Check sheet for the modelled part. Datum: model origin and axes. Units: mm. Face numbers are marked on the shaded views. A direction names the side the tool comes from. Round coordinates to 2 decimals unless told otherwise and drop trailing zeros. Order: outer loops, then holes, each group sorted by start corner. A loop starts at its lowest first (then second) coordinate and runs counter-clockwise, first axis right, second up.
```python
from build123d import *

# Parameters (mm, degrees)
BOX031_W                 = 46
BOX031_H                 = 15
BOX031_DEPTH             = 16
BOX029_W                 = 78
BOX029_H                 = 15
BOX029_DEPTH             = 6
BOX023_W                 = 220
BOX023_H                 = 2.5
BOX023_DEPTH             = 3
EXTRUDE011_DEPTH         = 10
BOX024_W                 = 220
BOX024_H                 = 113
BOX024_DEPTH             = 8
BOX026_W                 = 32
BOX026_H                 = 6
BOX026_DEPTH             = 6
PRISM004_DEPTH           = 6
PRISM004_PLACEMENT_ANGLE = 30
PRISM005_DEPTH           = 6
PRISM005_PLACEMENT_ANGLE = 30
EXTRUDE012_DEPTH         = 12.5
EXTRUDE009_DEPTH         = 12.5
EXTRUDE008_DEPTH         = 12.5
BOX009_W                 = 12.5
BOX009_H                 = 7.5
BOX009_DEPTH             = 22
BOX010_W                 = 12.5
BOX010_H                 = 7.5
BOX010_DEPTH             = 22
CYLINDER_R               = 1.7
CYLINDER_DEPTH           = 30
BOX007_W                 = 15
BOX007_H                 = 70
BOX007_DEPTH             = 6
BOX006_W                 = 40
BOX006_H                 = 51
BOX006_DEPTH             = 6
EXTRUDE010_DEPTH         = 12.5
BOX021_W                 = 12.5
BOX021_H                 = 7.5
BOX021_DEPTH             = 22
BOX027_W                 = 12.5
BOX027_H                 = 7.5
BOX027_DEPTH             = 22
CYLINDER002_R            = 1.7
CYLINDER002_DEPTH        = 30
BOX025_W                 = 15
BOX025_H                 = 70
BOX025_DEPTH             = 6
BOX022_W                 = 40
BOX022_H                 = 51
BOX022_DEPTH             = 6
BOX005_W                 = 20
BOX005_H                 = 6
BOX005_DEPTH             = 30
BOX004_W                 = 40
BOX004_H                 = 6
BOX004_DEPTH             = 44.5


with BuildPart() as cube030:
    # Box031 → Box031 (new body)
    with BuildSketch(Plane(origin=(-22, 15, 0), x_dir=(1, 0, 0), z_dir=(0, 0, 1))):
        with Locations((23, 7.5)):
            Rectangle(BOX031_W, BOX031_H)
    extrude(amount=BOX031_DEPTH)


with BuildPart() as cube028:
    # Box029 → Box029 (new body)
    with BuildSketch(Plane(origin=(-39, 0, 0), x_dir=(1, 0, 0), z_dir=(0, 0, 1))):
        with Locations((39, 7.5)):
            Rectangle(BOX029_W, BOX029_H)
    extrude(amount=BOX029_DEPTH)


with BuildPart() as cube022:
    # Box023 → Box023 (new body)
    with BuildSketch(Plane(origin=(-110, 2, 0), x_dir=(1, 0, 0), z_dir=(0, 0, 1))):
        with Locations((110, 1.25)):
            Rectangle(BOX023_W, BOX023_H)
    extrude(amount=BOX023_DEPTH)


with BuildPart() as extrude011:
    # Sketch009 → Extrude011 (new body)
    with BuildSketch(Plane.XY):
        Polygon((-95, 0), (95, 0), (85, 61), (-85, 61), align=None)
    extrude(amount=EXTRUDE011_DEPTH)


with BuildPart() as obj1:
    # Box024 → Box024 (new body)
    with BuildSketch(Plane(origin=(-110, -15, 0), x_dir=(1, 0, 0), z_dir=(0, 0, 1))):
        with Locations((110, 56.5)):
            Rectangle(BOX024_W, BOX024_H)
    extrude(amount=BOX024_DEPTH)

    # Cut004020: cut Extrude011
    add(extrude011.part, mode=Mode.SUBTRACT)


with BuildPart() as cube025:
    # Box026 → Box026 (new body)
    with BuildSketch(Plane(origin=(-16, 55, 0), x_dir=(1, 0, 0), z_dir=(0, 0, 1))):
        with Locations((16, 3)):
            Rectangle(BOX026_W, BOX026_H)
    extrude(amount=BOX026_DEPTH)


with BuildPart() as prism004:
    # Prism004 → Prism004 (new body)
    with BuildSketch(Plane.XY):
        Polygon((45, 0), (-22.5, 38.971143), (-22.5, -38.971143), align=None)
    extrude(amount=PRISM004_DEPTH)


with BuildPart() as prism004_1:
    # Prism004 placement: moved
    add(prism004.part.moved(Location((0, 23, 0))).rotate(Axis((0, 23, 0), (0, 0, -1)), PRISM004_PLACEMENT_ANGLE))


with BuildPart() as obj2:
    # Prism005 → Prism005 (new body)
    with BuildSketch(Plane.XY):
        Polygon((60, 0), (-30, 51.961524), (-30, -51.961524), align=None)
    extrude(amount=PRISM005_DEPTH)


with BuildPart() as obj2_1:
    # Prism005 placement: moved
    add(obj2.part.moved(Location((0, 23, 0))).rotate(Axis((0, 23, 0), (0, 0, -1)), PRISM005_PLACEMENT_ANGLE))

    # Cut004019: cut Prism004
    add(prism004_1.part, mode=Mode.SUBTRACT)


with BuildPart() as obj2_2:
    # Cut004019 placement: moved
    add(obj2_1.part.moved(Location((0, 7, 0))))

    # Fusion004005: union Cube025
    add(cube025.part)

    # Cut004015: cut obj1
    add(obj1.part, mode=Mode.SUBTRACT)

    # Cut004016: cut Cube022
    add(cube022.part, mode=Mode.SUBTRACT)


with BuildPart() as extrude012:
    # Sketch010 (on Face21 of Fusion004006) → Extrude012 (new body)
    with BuildSketch(Plane(origin=(-20, 0, 0), x_dir=(0, -1, 0), z_dir=(-1, 0, 0))):
        Polygon((-7.5, 0), (-7.5, 25), (-21.933757, 0), align=None)
    extrude(amount=-EXTRUDE012_DEPTH)


with BuildPart() as extrude012_1:
    # Extrude012 placement: moved
    add(extrude012.part.moved(Location((27.5, 0, 0))))


with BuildPart() as extrude009:
    # Sketch007 (on Face17 of Fusion004002) → Extrude009 (new body)
    with BuildSketch(Plane(origin=(-20, 0, 0), x_dir=(0, -1, 0), z_dir=(-1, 0, 0))):
        Polygon((0, 0), (0, 19), (45, 19), align=None)
    extrude(amount=EXTRUDE009_DEPTH)


with BuildPart() as extrude009_1:
    # Extrude009 placement: moved
    add(extrude009.part.moved(Location((40, 0, 0))))


with BuildPart() as extrude008:
    # Sketch007 (on Face17 of Fusion004002) → Extrude008 (new body)
    with BuildSketch(Plane(origin=(-20, 0, 0), x_dir=(0, -1, 0), z_dir=(-1, 0, 0))):
        Polygon((0, 0), (0, 19), (45, 19), align=None)
    extrude(amount=-EXTRUDE008_DEPTH)


with BuildPart() as cube008:
    # Box009 → Box009 (new body)
    with BuildSketch(Plane(origin=(7.5, 0, 3), x_dir=(1, 0, 0), z_dir=(0, 0, 1))):
        with Locations((6.25, 3.75)):
            Rectangle(BOX009_W, BOX009_H)
    extrude(amount=BOX009_DEPTH)


with BuildPart() as cube009:
    # Box010 → Box010 (new body)
    with BuildSketch(Plane(origin=(-20, 0, 3), x_dir=(1, 0, 0), z_dir=(0, 0, 1))):
        with Locations((6.25, 3.75)):
            Rectangle(BOX010_W, BOX010_H)
    extrude(amount=BOX010_DEPTH)


with BuildPart() as cylinder:
    # Cylinder → Cylinder (new body)
    with BuildSketch(Plane(origin=(0, 7, 0), x_dir=(1, 0, 0), z_dir=(0, 0, 1))):
        Circle(CYLINDER_R)
    extrude(amount=CYLINDER_DEPTH)


with BuildPart() as cube007:
    # Box007 → Box007 (new body)
    with BuildSketch(Plane(origin=(12.5, 22, 20), x_dir=(1, 0, 0), z_dir=(0, 0, 1))):
        with Locations((7.5, 35)):
            Rectangle(BOX007_W, BOX007_H)
    extrude(amount=BOX007_DEPTH)


with BuildPart() as fusion004002:
    # Box006 → Box006 (new body)
    with BuildSketch(Plane.XY.offset(20)):
        with Locations((20, 25.5)):
            Rectangle(BOX006_W, BOX006_H)
    extrude(amount=BOX006_DEPTH)

    # Cut004005: cut Cube007
    add(cube007.part, mode=Mode.SUBTRACT)


with BuildPart() as fusion004002_1:
    # Cut004005 placement: moved
    add(fusion004002.part.moved(Location((-20, 0, -1))))

    # Cut004006: cut Cylinder
    add(cylinder.part, mode=Mode.SUBTRACT)


with BuildPart() as fusion004002_2:
    # Cut004006 placement: moved
    add(fusion004002_1.part.moved(Location((0, -45, 0))))

    # Fusion004002: union Cube008, Cube009
    add(cube008.part)
    add(cube009.part)


with BuildPart() as fusion004007:
    # Sketch008 (on Face21 of Fusion004002) → Extrude010 (new body)
    with BuildSketch(Plane(origin=(-20, 0, 0), x_dir=(0, -1, 0), z_dir=(-1, 0, 0))):
        Polygon((-7.5, 0), (-7.5, 25), (-21.933757, 0), align=None)
    extrude(amount=-EXTRUDE010_DEPTH)

    # Fusion004007: union Extrude012, Extrude009, Extrude008, Fusion004002
    add(extrude012_1.part)
    add(extrude009_1.part)
    add(extrude008.part)
    add(fusion004002_2.part)


with BuildPart() as cube020:
    # Box021 → Box021 (new body)
    with BuildSketch(Plane(origin=(7.5, 0, 3), x_dir=(1, 0, 0), z_dir=(0, 0, 1))):
        with Locations((6.25, 3.75)):
            Rectangle(BOX021_W, BOX021_H)
    extrude(amount=BOX021_DEPTH)


with BuildPart() as cube026:
    # Box027 → Box027 (new body)
    with BuildSketch(Plane(origin=(-20, 0, 3), x_dir=(1, 0, 0), z_dir=(0, 0, 1))):
        with Locations((6.25, 3.75)):
            Rectangle(BOX027_W, BOX027_H)
    extrude(amount=BOX027_DEPTH)


with BuildPart() as cylinder002:
    # Cylinder002 → Cylinder002 (new body)
    with BuildSketch(Plane(origin=(0, 7, 0), x_dir=(1, 0, 0), z_dir=(0, 0, 1))):
        Circle(CYLINDER002_R)
    extrude(amount=CYLINDER002_DEPTH)


with BuildPart() as cube024:
    # Box025 → Box025 (new body)
    with BuildSketch(Plane(origin=(12.5, 22, 20), x_dir=(1, 0, 0), z_dir=(0, 0, 1))):
        with Locations((7.5, 35)):
            Rectangle(BOX025_W, BOX025_H)
    extrude(amount=BOX025_DEPTH)


with BuildPart() as parte_frontal:
    # Box022 → Box022 (new body)
    with BuildSketch(Plane.XY.offset(20)):
        with Locations((20, 25.5)):
            Rectangle(BOX022_W, BOX022_H)
    extrude(amount=BOX022_DEPTH)

    # Cut004017: cut Cube024
    add(cube024.part, mode=Mode.SUBTRACT)


with BuildPart() as parte_frontal_1:
    # Cut004017 placement: moved
    add(parte_frontal.part.moved(Location((-20, 0, -1))))

    # Cut004018: cut Cylinder002
    add(cylinder002.part, mode=Mode.SUBTRACT)


with BuildPart() as parte_frontal_2:
    # Cut004018 placement: moved
    add(parte_frontal_1.part.moved(Location((0, -45, 0))))

    # Fusion004006: union Cube020, Cube026
    add(cube020.part)
    add(cube026.part)

    # Fusion004008: union Fusion004007
    add(fusion004007.part)


with BuildPart() as cube005:
    # Box005 → Box005 (new body)
    with BuildSketch(Plane(origin=(-10, 55, 6), x_dir=(1, 0, 0), z_dir=(0, 0, 1))):
        with Locations((10, 3)):
            Rectangle(BOX005_W, BOX005_H)
    extrude(amount=BOX005_DEPTH)


with BuildPart() as cut004022:
    # Box004 → Box004 (new body)
    with BuildSketch(Plane(origin=(-20, 55, 0), x_dir=(1, 0, 0), z_dir=(0, 0, 1))):
        with Locations((20, 3)):
            Rectangle(BOX004_W, BOX004_H)
    extrude(amount=BOX004_DEPTH)

    # Cut004004: cut Cube005
    add(cube005.part, mode=Mode.SUBTRACT)

    # Fusion004009: union obj2, parte_frontal
    add(obj2_2.part)
    add(parte_frontal_2.part)

    # Fusion004009002: union Cube028
    add(cube028.part)

    # Cut004022: cut Cube030
    add(cube030.part, mode=Mode.SUBTRACT)


solid = cut004022.part
```
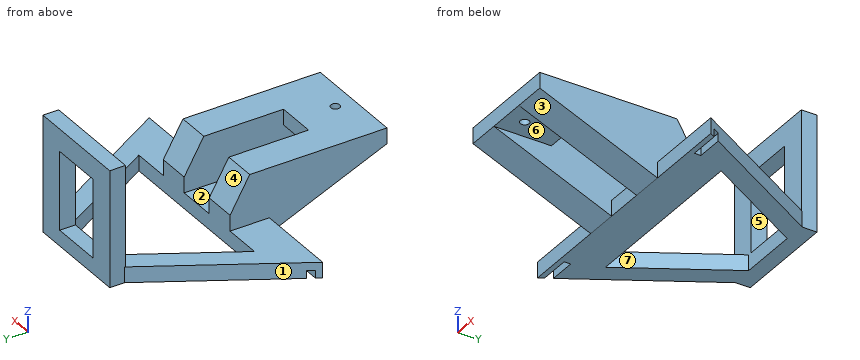
Item 1: Sectioned sample at B-B (z = 30). Record the cut outline in (x, y).
Answer:
outline: (-20, 55) - (-10, 55) - (-10, 61) - (-20, 61) - close; (10, 55) - (20, 55) - (20, 61) - (10, 61) - close
Item 2: Sectioned sample at A-A (x = 0). Record the cut outline in (y, z).
Answer:
outline: (-45, 19) - (-39.7, 19) - (-39.7, 25) - (-45, 25) - close; (-36.3, 19) - (-23, 19) - (-23, 25) - (-36.3, 25) - close; (0, 0) - (15, 0) - (15, 6) - (0, 6) - close; (55, 0) - (61, 0) - (61, 6) - (55, 6) - close; (55, 36) - (61, 36) - (61, 44.5) - (55, 44.5) - close
Item 3: Go/stop test with flat-tipped pins: P1, Ø4, axis at x = -2, y = 12, coming from the +Z side; P2, Ø7.5, axis at y = -3, z = 9, coming from the +X side; P3, Ø2, axis at x = -0.5, y = 16.5, coming from the -Z side; P4, Ø12.5, axis at y = -14.5, z = 14, coming from the -X side. Record where each tip stops, or that it passes through.
Answer:
P1: stops at z = 6
P2: stops at x = 20
P3: passes through
P4: stops at x = -20
Item 4: Release check for a two-part mould opening along X. For the marked faces 1, 2 and 3 record: released by +X, released by -X, zero draft, split by the parting line, or undercut.
Answer:
face 1: released by -X
face 2: undercut
face 3: zero draft
Item 5: Access from +Z, -Z, +X, -X, +Y, -Y to the whole of each face (thin tool, end or side, straight path). Record for the marked faces 4, 5, 6 and 7.
Answer:
face 4: +Z, +X, -X
face 5: +Y
face 6: -Z, +Y, -Y
face 7: +Z, -Z
Item 6: Scan lines: line 1 along Y through (x, z) = (0, 22.25); line 2 along X through (y, z) = (-38, 22); line 3 along Y through (x, z) = (19, 26). Record each from-to range of solid material in increasing order.
Answer:
line 1: y = -45 to -39.7, -36.3 to -23
line 2: x = -20 to -1.7, 1.7 to 20
line 3: y = 55 to 61
Item 7: Sectioned sample at C-C (z = 23). Record the cut outline in (x, y), and give its area (3 significant figures).
Answer:
outline: (-20, -45) - (20, -45) - (20, 8.65) - (7.5, 8.65) - (7.5, -23) - (-7.5, -23) - (-7.5, 8.65) - (-20, 8.65) - close; (-20, 55) - (-10, 55) - (-10, 61) - (-20, 61) - close; (10, 55) - (20, 55) - (20, 61) - (10, 61) - close; hole circle Ø3.4 at (0, -38)
area: 1,780 mm2
Item 8: Sectioned sample at D-D (y = -38). Record the cut outline in (x, z), and give its area (3 significant figures).
Answer:
outline: (-20, 16.04) - (-7.5, 16.04) - (-7.5, 19) - (-1.7, 19) - (-1.7, 25) - (-20, 25) - close; (1.7, 19) - (7.5, 19) - (7.5, 16.04) - (20, 16.04) - (20, 25) - (1.7, 25) - close
area: 293 mm2
